Design review of the part built by this model. Coordinates are the model's own, in mm. Coordinates: 2 decimals unless noted, no trailing zeros. Loops run counter-clockwise (first coordinate to the right, second up) from the corner with the lowest first, then second, coordinate; pieces in that order, holes last. Notation, with made-up numbers: (54.5, 70) -> (63.5, 70) arc R11 ccw to (63.5, 77) -> close; hole circle Ø5 at (39, -27). An arc over 180 degrees is marked (long way). Answer in a Markdown table with one row per item.
```python
from build123d import *

# Parameters (mm, degrees)
SKETCH1_R           = 13.335
BOSS_EXTRUDE1_DEPTH = 3.175
SKETCH2_R           = 3.175
SKETCH2_R_2         = 1.5875
CUT_EXTRUDE1_DEPTH  = 74.369297053
EDGE_FLANGE2_DEPTH  = 69.85


# Sheet-metal steps are written as plain solids
with BuildPart() as part:
    # Sketch1 → Boss-Extrude1 (new body)
    with BuildSketch(Plane(origin=(0, 0, 0), x_dir=(1, 0, 0), z_dir=(0, 1, 0))):
        with BuildLine():
            Line((22.225, 0), (22.225, 69.85))
            Line((22.225, 69.85), (-22.225, 69.85))
            Line((-22.225, 69.85), (-22.225, 0))
            ThreePointArc((-22.225, 0), (0, -22.225), (22.225, 0))
        make_face()
        with Locations(Location((0, 0, 0), (0, 0, 270))):
            Circle(SKETCH1_R, mode=Mode.SUBTRACT)
    extrude(amount=BOSS_EXTRUDE1_DEPTH)

    # Sketch2 → Cut-Extrude1 (cut, through all)
    with BuildSketch(Plane(origin=(0, 3.175, 0), x_dir=(1, 0, 0), z_dir=(0, 1, 0))):
        with Locations(Location((-12.7, 57.15, 0), (0, 0, 270))):
            Circle(SKETCH2_R)
        with Locations(Location((12.7, 57.15, 0), (0, 0, 270))):
            Circle(SKETCH2_R)
        with Locations(Location((0, 15.494, 0), (0, 0, 270))):
            Circle(SKETCH2_R_2)
        with Locations(Location((5.299260101, 14.559597466, 0), (0, 0, 270))):
            Circle(SKETCH2_R_2)
        with Locations(Location((9.959351224, 11.869092602, 0), (0, 0, 270))):
            Circle(SKETCH2_R_2)
        with Locations(Location((13.418197606, 7.747, 0), (0, 0, 270))):
            Circle(SKETCH2_R_2)
        with Locations(Location((15.258611325, 2.690504865, 0), (0, 0, 270))):
            Circle(SKETCH2_R_2)
        with Locations(Location((15.258611325, -2.690504865, 0), (0, 0, 270))):
            Circle(SKETCH2_R_2)
        with Locations(Location((13.418197606, -7.747, 0), (0, 0, 270))):
            Circle(SKETCH2_R_2)
        with Locations(Location((9.959351224, -11.869092602, 0), (0, 0, 270))):
            Circle(SKETCH2_R_2)
        with Locations(Location((5.299260101, -14.559597466, 0), (0, 0, 270))):
            Circle(SKETCH2_R_2)
        with Locations(Location((0, -15.494, 0), (0, 0, 270))):
            Circle(SKETCH2_R_2)
        with Locations(Location((-5.299260101, -14.559597466, 0), (0, 0, 270))):
            Circle(SKETCH2_R_2)
        with Locations(Location((-9.959351224, -11.869092602, 0), (0, 0, 270))):
            Circle(SKETCH2_R_2)
        with Locations(Location((-13.418197606, -7.747, 0), (0, 0, 270))):
            Circle(SKETCH2_R_2)
        with Locations(Location((-15.258611325, -2.690504865, 0), (0, 0, 270))):
            Circle(SKETCH2_R_2)
        with Locations(Location((-15.258611325, 2.690504865, 0), (0, 0, 270))):
            Circle(SKETCH2_R_2)
        with Locations(Location((-13.418197606, 7.747, 0), (0, 0, 270))):
            Circle(SKETCH2_R_2)
        with Locations(Location((-9.959351224, 11.869092602, 0), (0, 0, 270))):
            Circle(SKETCH2_R_2)
        with Locations(Location((-5.299260101, 14.559597466, 0), (0, 0, 270))):
            Circle(SKETCH2_R_2)
    extrude(amount=-CUT_EXTRUDE1_DEPTH, mode=Mode.SUBTRACT)

    # Edge-Flange2 section (across the edge) → Edge-Flange2 (add)
    with BuildSketch(Plane(origin=(22.733, 3.175, 0), x_dir=(-1, 0, 0), z_dir=(0, 0, -1))):
        with BuildLine():
            Line((-3.175, 0.508), (-3.175, 3.175))
            Line((-3.175, 3.175), (0, 3.175))
            Line((0, 3.175), (0, 0.508))
            ThreePointArc((0, 0.508), (0.148789755, 0.148789755), (0.508, 0))
            Line((0.508, 0), (0.508, -3.175))
            ThreePointArc((0.508, -3.175), (-2.096274275, -2.096274275), (-3.175, 0.508))
        make_face()
    extrude(amount=EDGE_FLANGE2_DEPTH)


solid = part.part
```
(1) Draft analysis for pull direction Z (two halves, no side actions). For faces 1 (the flat face through (24, 3, 0)), 2 (the flat face through (22.733, 5, -34)), 3 (the cylindrical face through (5.369, 1.61, -16.146)), 4 (the flat face through (2, 2, -69.85)), state which applies: pulls with the +Z half, pulls with the -Z half, needs draft (parallel to the pull), parting line crosses it, or undercut.
Evaluation:
| item | result |
|---|---|
| face 1 | pulls with the +Z half |
| face 2 | needs draft |
| face 3 | undercut |
| face 4 | pulls with the -Z half |
(2) Take a section at D-D on x = -18. Give the boundary of the cut face in (y, z) (3 decimals), and give its area (3 significant figures).
Evaluation:
| item | result |
|---|---|
| outline | (0, -69.85) -> (3.175, -69.85) -> (3.175, 13.037) -> (0, 13.037) -> close |
| area | 263 mm² |
(3) Take a section at C-C on z = -18.5. Give the boundary of the cut face in (x, y) (3 decimals).
Evaluation:
| item | result |
|---|---|
| outline | (-22.225, 0) -> (22.225, 0) arc R3.683 ccw to (25.908, 3.683) -> (25.908, 6.35) -> (22.733, 6.35) -> (22.733, 3.683) arc R0.508 cw to (22.225, 3.175) -> (-22.225, 3.175) -> close |
(4) For pin 1 (4 mm diameter, centred on x = 9.96, z = 11.87, fed in from +Y) (3 decimals); pin 2 (2 mm diameter, centred on x = 3, y = 3, fed in from +Z); pin 3 (4 mm diameter, centred on x = -9.96, z = -11.87, fed in from -Y); pin 4 (2 mm diameter, centred on y = 1.5, z = -5, fed in from +X), all flat-tipped, find the tip position at first contact; note any pin that passes through.
Evaluation:
| item | result |
|---|---|
| pin 1 | stops at y = 3.175 |
| pin 2 | stops at z = 22.13 |
| pin 3 | stops at y = 0 |
| pin 4 | stops at x = 25.71 |
(5) Take a section at A-A on z = -57.15. Give the boundary of the cut face in (x, y) (3 decimals), and give its area (3 significant figures).
Evaluation:
| item | result |
|---|---|
| outline | (-22.225, 0) -> (-15.875, 0) -> (-15.875, 3.175) -> (-22.225, 3.175) -> close; (-9.525, 0) -> (9.525, 0) -> (9.525, 3.175) -> (-9.525, 3.175) -> close; (15.875, 0) -> (22.225, 0) arc R3.683 ccw to (25.908, 3.683) -> (25.908, 6.35) -> (22.733, 6.35) -> (22.733, 3.683) arc R0.508 cw to (22.225, 3.175) -> (15.875, 3.175) -> close |
| area | 120 mm² |
(6) Take a section at B-B on z = -7. Give the boundary of the cut face in (x, y) (3 decimals).
Evaluation:
| item | result |
|---|---|
| outline | (-22.225, 0) -> (-14.819, 0) -> (-14.819, 3.175) -> (-22.225, 3.175) -> close; (-12.017, 0) -> (-11.35, 0) -> (-11.35, 3.175) -> (-12.017, 3.175) -> close; (11.35, 0) -> (12.017, 0) -> (12.017, 3.175) -> (11.35, 3.175) -> close; (14.819, 0) -> (22.225, 0) arc R3.683 ccw to (25.908, 3.683) -> (25.908, 6.35) -> (22.733, 6.35) -> (22.733, 3.683) arc R0.508 cw to (22.225, 3.175) -> (14.819, 3.175) -> close |
(7) To check wall thickness, follow probe 1 along X at (y, z) = (2.5, -59) (3 decimals); probe 2 along X at (y, z) = (2, 9); probe 3 along X at (y, z) = (1.65, -57.15) (3 decimals). State the ranges of each line that lie inside material, in increasing order.
Evaluation:
| item | result |
|---|---|
| probe 1 | x = -22.225 to -15.28, -10.12 to 10.12, 15.28 to 25.713 |
| probe 2 | x = -20.32 to -14.39, -12.44 to -9.84, 9.84 to 12.44, 14.39 to 20.32 |
| probe 3 | x = -22.225 to -15.875, -9.525 to 9.525, 15.875 to 25.296 |
